Source: CAD feature listing. Evaluate the final solid. Frame: model axes, mm. A direction names the side the tool comes from. Give positions to 0.01 mm unless a question says otherwise; leave off trailing zeros. Order: outer loops, then holes, each group sorted by start corner. A loop starts at its lowest first (then second) coordinate and runs counter-clockwise, first axis right, second up. Notation, with made-up numbers: M 30.5,16 L 51.5,16 A14 cw 51.5,30 Z; hole C 52.25,54.5 d2. An arc over 180 degrees is marked long. Answer as a JSON object with one key per item and string values. Group by question number.
1. Section query C-C (x = -18). Output: boundary loops of the cut face in (y, z) (3 decimals), plus the area to 3 significant figures.
2. Pin query (flat end, axial travel): P1, Ø20.5, axis at x = -1.1, z = -59.55, coming from the -Y side; P2, Ø5, axis at y = -3, z = -1, coming from the -X side; P3, Ø1.5, axis at y = -14, z = -11.5, coming from the +X side; P4, Ø4, axis at y = -7, z = -10.5, coming from the +X side. Return the tip coordinate at first contact, or that it passes through.
3. Section query A-A (y = -4). Count the separate pieces of the cut face and the enclosed holes in it, plus the area to 3 significant figures.
4. Material intervals for L1, parallel to Z at x = -6.5, y = -6.25; L2, parallel to Z at x = 4, y = -16.75; L3, parallel to Z at x = -1.5, y = -12, sorted ascending. Write a range as [from, to].
5. Set-up query: faces 4 (the flat face through (-17.8, -0.3, 4.7)), 5 (the cylindrical face through (-1.793, -12.624, 21.45)). Return all of +Z, -Z, +X, -X, +Y, -Y with unobstructed straight access to the full face (end or side cutting, diameter ignored); none if empty.
6. Section query B-B (z = -15). Output: boundary loops of the cut face in (x, y) (3 decimals).
7. Pull-direction query (Z, two-part tool) for faces 1 (the flat face through (15.856, -18.686, 4.046)), 2 (the flat face through (-26.504, -9, -47)), 3 (the cylindrical face through (-3.17, -9.61, -1.56)); classes: +Z half, -Z half, draft (parallel to the pull), parting line (faces both ways), or undercut.
from build123d import *

# Parameters (mm, degrees)
F1_DEPTH = 18.9992
F2_R     = 9.525
F3_DEPTH = 25.4
F4_R     = 6.35
F5_DEPTH = 25.4
F6_R     = 3.175
F7_DEPTH = 12.7
F8_SIZE2 = 1.27
F8_SIZE  = 1.27
F9_SIZE  = 0.635


with BuildPart() as f1:
    # F0 (on Front) → F1 (new body)
    with BuildSketch(Plane.XZ):
        Polygon((7.785652, 26.052904), (-9.994348, 26.052904), (-26.504348, -17.127096), (-26.504348, -78.087096), (24.295652, -78.087096), (24.295652, -17.127096), align=None)
    extrude(amount=F1_DEPTH)

    # F2 (on face) → F3 (cut)
    with BuildSketch(Plane.XZ.offset(18.9992)):
        with Locations((-1.104348, 7.739504)):
            Circle(F2_R)
    extrude(amount=-F3_DEPTH, mode=Mode.SUBTRACT)

    # F4 (on face) → F5 (cut)
    with BuildSketch(Plane.XZ.offset(18.9992)):
        with Locations((-1.104348, -59.545096)):
            Circle(F4_R)
    extrude(amount=-F5_DEPTH, mode=Mode.SUBTRACT)

    # F6 (on face) → F7 (cut)
    with BuildSketch(Plane.XY.offset(26.052904)):
        with Locations((-1.104348, -9.525)):
            Circle(F6_R)
    extrude(amount=-F7_DEPTH, mode=Mode.SUBTRACT)

    # F8
    f8_edges = [f1.edges().sort_by_distance(p)[0] for p in [
        (-10.629348, -18.9992, 7.739504),
        (-7.454348, -18.9992, -59.545096),
        (-10.629348, 0, 7.739504),
        (-7.454348, 0, -59.545096),
    ]]
    chamfer(f8_edges, length=F8_SIZE, length2=F8_SIZE2)

    # F9
    f9_edges = [f1.edges().sort_by_distance(p)[0] for p in [
        (-18.249348, 0, 4.462904),
        (-26.504348, 0, -47.607096),
        (-1.104348, 0, -78.087096),
        (24.295652, 0, -47.607096),
        (16.040652, 0, 4.462904),
        (-1.104348, 0, 26.052904),
        (-26.504348, -18.9992, -47.607096),
        (-1.104348, -18.9992, -78.087096),
        (24.295652, -18.9992, -47.607096),
        (16.040652, -18.9992, 4.462904),
        (-1.104348, -18.9992, 26.052904),
        (-18.249348, -18.9992, 4.462904),
    ]]
    chamfer(f9_edges, length=F9_SIZE)


solid = f1.part
Answer sheet:
{
 "1": {"outline": "M -18.999,-77.452 L -18.364,-78.087 L -0.635,-78.087 L 0,-77.452 L 0,3.337 L -0.635,5.115 L -18.364,5.115 L -18.999,3.337 Z", "area": "1,580 mm^2"},
 "2": {"P1": "y = -19", "P2": "x = -21.29", "P3": "x = 22.43", "P4": "x = 22.53"},
 "3": {"separate pieces": "1", "enclosed holes": "2", "area": "4,170 mm^2"},
 "4": {"L1": "[-78.09, -62.89], [-56.2, -0.11], [15.59, 26.05]", "L2": "[-78.09, -63.32], [-55.77, -0.3], [15.78, 26.05]", "L3": "[-78.09, -65.88], [-53.21, -1.78]"},
 "5": {"face 4": "+Z, -X, +Y", "face 5": "+Z"},
 "6": {"outline": "M -25.691,-18.364 L -25.011,-18.999 L 22.803,-18.999 L 23.482,-18.364 L 23.482,-0.635 L 22.803,0 L -25.011,0 L -25.691,-0.635 Z"},
 "7": {"face 1": "+Z half", "face 2": "draft", "face 3": "undercut"}
}
